Build history of the part. All positions in model axes, mm. A direction names the side the tool comes from. Coordinates: 2 decimals unless noted, no trailing zeros. Order: outer loops, then holes, each group sorted by start corner. A loop starts at its lowest first (then second) coordinate and runs counter-clockwise, first axis right, second up. Notation, with made-up numbers: (0.5, 27) - (8.5, 27) arc R23 cw to (8.5, 47) - close; hole circle Ø6 at (29, -5.5). An arc over 180 degrees is marked (long way). Return JSON: item names as keys, results as strings.
from build123d import *

# Parameters (mm, degrees)
AUFSATZ_LINEAR_AUSTRAGEN1_DEPTH      = 35
SCHNITT_LINEAR_AUSTRAGEN1_DEPTH      = 85.150163399
SCHNITT_LINEAR_AUSTRAGEN1_DEPTH_BACK = 85.150163399
FASE6_SIZE                           = 3
FASE6_SIZE2                          = 5.591073264
FASE6_EDGE_2_SIZE                    = 3
FASE6_EDGE_2_SIZE2                   = 5.591073264
FASE7_SIZE                           = 10
WANDUNG3_T                           = -2
SCHNITT_LINEAR_AUSTRAGEN2_REACH      = 86.15
SKIZZE9_W                            = 10
SKIZZE9_H                            = 35
SKIZZE10_R                           = 1.6
AUFSATZ_LINEAR_AUSTRAGEN3_DEPTH      = 10
VERRUNDUNG4_R                        = 1


with BuildPart() as part:
    # Skizze6 → Aufsatz-Linear austragen1 (new body)
    with BuildSketch(Plane(origin=(0, 0, 0), x_dir=(1, 0, 0), z_dir=(0, 1, 0))):
        Polygon((30, -35), (-30, -35), (-47.5, -20), (-47.5, 25), (-20, 60), (20, 60), (47.5, 25), (47.5, -20), align=None)
    extrude(amount=AUFSATZ_LINEAR_AUSTRAGEN1_DEPTH)

    # Skizze8 → Schnitt-Linear austragen1 (cut, two sides: drawn at the far end of the back side and taken through both)
    with BuildSketch(Plane(origin=(0, 0, 0), x_dir=(0, 0, -1), z_dir=(1, 0, 0)).offset(-SCHNITT_LINEAR_AUSTRAGEN1_DEPTH_BACK)):
        Polygon((20, 35), (60, 3), (60, 35), align=None)
    extrude(amount=SCHNITT_LINEAR_AUSTRAGEN1_DEPTH + SCHNITT_LINEAR_AUSTRAGEN1_DEPTH_BACK, mode=Mode.SUBTRACT)

    # Fase6
    fase6_edges = [part.edges().sort_by_distance(p)[0] for p in [
        (33.75, 17, -42.5),
    ]]
    fase6_side = [part.faces().sort_by_distance(p)[0] for p in [
        (0, 21.261380323, -37.173274596),
    ]]
    chamfer(fase6_edges, length=FASE6_SIZE, length2=FASE6_SIZE2, reference=fase6_side[0])

    # Fase6 edge 2
    fase6_edge_2_edges = [part.edges().sort_by_distance(p)[0] for p in [
        (-33.75, 17, -42.5),
    ]]
    fase6_edge_2_side = [part.faces().sort_by_distance(p)[0] for p in [
        (0, 21.261380323, -37.173274596),
    ]]
    chamfer(fase6_edge_2_edges, length=FASE6_EDGE_2_SIZE, length2=FASE6_EDGE_2_SIZE2, reference=fase6_edge_2_side[0])

    # Fase7
    fase7_edges = [part.edges().sort_by_distance(p)[0] for p in [
        (0, 35, 35),
    ]]
    chamfer(fase7_edges, length=FASE7_SIZE)

    # Wandung3
    wandung3_openings = [part.faces().sort_by_distance(p)[0] for p in [
        (0, 35, 2.356885836),
    ]]
    offset(amount=WANDUNG3_T, openings=wandung3_openings, kind=Kind.INTERSECTION)

    # Skizze9 → Schnitt-Linear austragen2 (cut, up to next)
    with BuildSketch(Plane.XZ, mode=Mode.PRIVATE) as schnitt_linear_austragen2_sk1:
        with Locations((-35, 2)):
            Rectangle(SKIZZE9_W, SKIZZE9_H)
    schnitt_linear_austragen2_tool1 = extrude(schnitt_linear_austragen2_sk1.sketch, amount=-SCHNITT_LINEAR_AUSTRAGEN2_REACH, mode=Mode.PRIVATE) & part.part
    # Skizze9 → Schnitt-Linear austragen2 (cut, up to next)
    with BuildSketch(Plane.XZ, mode=Mode.PRIVATE) as schnitt_linear_austragen2_sk2:
        with Locations((35, 2)):
            Rectangle(SKIZZE9_W, SKIZZE9_H)
    schnitt_linear_austragen2_tool2 = extrude(schnitt_linear_austragen2_sk2.sketch, amount=-SCHNITT_LINEAR_AUSTRAGEN2_REACH, mode=Mode.PRIVATE) & part.part
    add(schnitt_linear_austragen2_tool1.solids().sort_by_distance((-35, 0, 2))[0], mode=Mode.SUBTRACT)
    add(schnitt_linear_austragen2_tool2.solids().sort_by_distance((35, 0, 2))[0], mode=Mode.SUBTRACT)

    # Skizze10 → Aufsatz-Linear austragen3 (add)
    # profile 1 of 2: a face of its own
    with BuildSketch(Plane(origin=(0, 2, 0), x_dir=(1, 0, 0), z_dir=(0, 1, 0))):
        with BuildLine():
            Line((-30, 4), (-27.645751311, 4))
            ThreePointArc((-27.645751311, 4), (-25, 11), (-22.354248689, 4))
            Line((-22.354248689, 4), (-20, 4))
            Line((-20, 4), (-20, -8))
            Line((-20, -8), (-22.354248689, -8))
            ThreePointArc((-22.354248689, -8), (-25, -15), (-27.645751311, -8))
            Line((-27.645751311, -8), (-30, -8))
            Line((-30, -8), (-30, 4))
        make_face()
        with Locations(Location((-25, 7, 0), (0, 0, 270))):
            Circle(SKIZZE10_R, mode=Mode.SUBTRACT)
        with Locations(Location((-25, -11, 0), (0, 0, 90))):
            Circle(SKIZZE10_R, mode=Mode.SUBTRACT)
    # profile 2 of 2: a face of its own
    with BuildSketch(Plane(origin=(0, 2, 0), x_dir=(1, 0, 0), z_dir=(0, 1, 0))):
        with BuildLine():
            Line((22.354248689, -8), (20, -8))
            Line((20, -8), (20, 4))
            Line((20, 4), (22.354248689, 4))
            ThreePointArc((22.354248689, 4), (25, 11), (27.645751311, 4))
            Line((27.645751311, 4), (30, 4))
            Line((30, 4), (30, -8))
            Line((30, -8), (27.645751311, -8))
            ThreePointArc((27.645751311, -8), (25, -15), (22.354248689, -8))
        make_face()
        with Locations(Location((25, -11, 0), (0, 0, 270))):
            Circle(SKIZZE10_R, mode=Mode.SUBTRACT)
        with Locations(Location((25, 7, 0), (0, 0, 90))):
            Circle(SKIZZE10_R, mode=Mode.SUBTRACT)
    extrude(amount=AUFSATZ_LINEAR_AUSTRAGEN3_DEPTH)

    # Verrundung4
    verrundung4_edges = [part.edges().sort_by_distance(p)[0] for p in [
        (-22.354248689, 7, 8),
        (-22.354248689, 7, -4),
        (-27.645751311, 7, -4),
        (-27.645751311, 7, 8),
        (27.645751311, 7, -4),
        (22.354248689, 7, -4),
        (22.354248689, 7, 8),
        (27.645751311, 7, 8),
    ]]
    fillet(verrundung4_edges, radius=VERRUNDUNG4_R)


solid = part.part
1. Drop flat-ended pins along their axis: pin 1 (1 mm diameter, centred on x = 34, y = 1.5, fed in from +Z); pin 2 (11 mm diameter, centred on x = 13.5, y = 18.5, fed in from -Z); pin 3 (8 mm diameter, centred on x = -25.5, z = 7, fed in from +Y). Give the stop position or say it passes through.
Check values:
{"pin 1": "z = 32", "pin 2": "z = -47.5", "pin 3": "y = 12"}
2. Mould opens along Y. For faces 1 (the flat face through (37.494, 18.269, 25.943)), 2 (the cylindrical face through (-25, 7, 15)), 3 (the flat face through (25, 2, -7)) say: pulls with the +Y half, pulls with the -Y half, needs draft (parallel to the pull), parting line crosses it, or undercut.
Check values:
{"face 1": "undercut", "face 2": "needs draft", "face 3": "pulls with the +Y half"}
3. Cut at B-B on y = 16.5. Give the cut face in (x, z) (3 decimals), plus the area to 3 significant figures.
Check values:
{"outline": "(-47.5, -25) - (-39.746, -34.868) - (-29.739, -43.125) - (29.739, -43.125) - (39.746, -34.868) - (47.5, -25) - (47.5, 20) - (30, 35) - (-30, 35) - (-47.5, 20) - close; hole (-45.5, -24.308) - (-38.631, -33.051) - (-30.301, -39.923) - (30.301, -39.923) - (38.631, -33.051) - (45.5, -24.308) - (45.5, 19.08) - (29.26, 33) - (-29.26, 33) - (-45.5, 19.08) - close", "area": "674 mm²"}
4. Cut at A-A on z = -7. State how many separate pieces and enclosed holes the cut face has, plus the area to 3 significant figures.
Check values:
{"separate pieces": "3", "enclosed holes": "0", "area": "378 mm²"}
5. Cut at D-D on x = -32. Give the cut face in (y, z), plus the area to 3 significant figures.
Check values:
{"outline": "(0, -44.73) - (8.61, -44.73) - (18.8, -40.25) - (35, -20) - (35, -16.8) - (18.23, -37.76) - (9.75, -41.49) - (2, -41.49) - (2, -15.5) - (0, -15.5) - close; (0, 19.5) - (2, 19.5) - (2, 30.65) - (26.52, 30.65) - (35, 22.17) - (35, 25) - (26.71, 33.29) - (0, 33.29) - close", "area": "276 mm²"}
6. Probe L1, parallel to X at y = 8, z = 5; L2, parallel to X at y = 6.75, z = 11; L3, parallel to X at y = 29.5, z = -17.5. List the from-to ranges inside material, lowest first.
Check values:
{"L1": "-47.5 to -45.5, -30 to -20, 20 to 30, 45.5 to 47.5", "L2": "-47.5 to -45.5, -29 to -26.6, -23.4 to -21, 21 to 23.4, 26.6 to 29, 45.5 to 47.5", "L3": "-47.5 to -45.5, 45.5 to 47.5"}
7. Tool access for faces 4 (the flat face through (-38.35, 9.316, -36.645)), 5 (the flat face through (-20, 7, 2)), 6 (the flat face through (-32.86, 14.8, -38.56)): list every direction of +Z, -Z, +X, -X, +Y, -Y with a clear straight run to the whole face (end or side of a thin tool).
Check values:
{"face 4": "-Z, -X, +Y, -Y", "face 5": "+Y", "face 6": "none"}
